Solid Edge part; units mm, degrees
sketch "Sketch1" plane through (0, 0, 0) normal (0, 0, 1) x (1, 0, 0)
  circle A0 centre (0, 0) radius 41.05
  circle A1 centre (0, 0) radius 20.625
  circle A2 centre (159.79, 0) radius 23.37
  circle A3 centre (159.79, 0) radius 13.21
extrude "Protrusion1" add sketch "Sketch1" along normal blind 17.73
sketch "Sketch2" plane through (0, 0, 0) normal (0, 0, 1) x (1, 0, 0)
  line L0 (159.79, -23.37) -> (139.6358, 0)
  line L1 (139.6358, 0) -> (159.79, 23.37)
  line L2 (8.6959, 40.1184) -> (159.79, 23.37)
  line L3 (8.6959, 40.1184) -> (28.7283, 0)
  line L4 (28.7283, 0) -> (8.6959, -40.1184)
  line L5 (159.79, -23.37) -> (8.6959, -40.1184)
extrude "ExtrudedProtrusion_2" add sketch "Sketch2" along normal blind 12.7
sketch "Sketch3" plane through (0, 0, 0) normal (0, 0, 1) x (1, 0, 0)
  line L0 (-5.0718, -15.3845) -> (-10.7875, -12.0845)
  line L1 (-10.7875, -12.0845) -> (-13.2875, -16.4147)
  line L2 (-13.2875, -16.4147) -> (-7.5718, -19.7147)
  line L3 (-5.0718, -15.3845) -> (-7.5718, -19.7147)
  line L4 (-10.7875, 12.0845) -> (-5.0718, 15.3845)
  line L5 (-5.0718, 15.3845) -> (-7.5718, 19.7147)
  line L6 (-7.5718, 19.7147) -> (-13.2875, 16.4147)
  line L7 (-10.7875, 12.0845) -> (-13.2875, 16.4147)
  line L8 (15.8593, -3.3) -> (20.8593, -3.3)
  line L9 (20.8593, -3.3) -> (20.8593, 3.3)
  line L10 (15.8593, 3.3) -> (20.8593, 3.3)
  line L11 (15.8593, 3.3) -> (15.8593, -3.3)
extrude "Protrusion2" add sketch "Sketch3" along normal up to vertex (17.73 mm away)
Verification items for the finished model (mm, model axes). A direction names the side the tool comes from. Give positions to 0.01 mm unless a question says otherwise; leave off trailing zeros. Loops run counter-clockwise (first coordinate to the right, second up) from the corner with the lowest first, then second, coordinate; pieces in that order, holes last.
1. Release check for a two-part mould opening along Y. For faces 1 (the flat face through (69, 1, 0)), 2 (the cylindrical face through (181.38, 8.95, 10.71)), 3 (the flat face through (-11.9, -14.01, 8.74)) record: +Y half, -Y half, draft (parallel to the pull), parting line (faces both ways), or undercut.
Derived:
face 1: draft
face 2: parting line
face 3: undercut
2. Material ranges on probe 1 along X at (y, z) = (-17, 14.5); probe 2 along X at (y, z) = (1.5, 11.25); probe 3 along Y at (x, z) = (159.79, 14.25), recorded low to high.
Derived:
probe 1: x = -37.36 to -6, 11.68 to 37.36, 143.75 to 175.83
probe 2: x = -41.02 to -20.57, 15.86 to 146.67, 172.91 to 183.11
probe 3: y = -23.37 to -13.21, 13.21 to 23.37
3. Cross-section at B-B on x = 0. Record the cut outline in (y, z) (3 decimals), and give its area (3 significant figures).
Derived:
outline: (-41.05, 0) - (-20.625, 0) - (-20.625, 17.73) - (-41.05, 17.73) - close; (20.625, 0) - (41.05, 0) - (41.05, 17.73) - (20.625, 17.73) - close
area: 724 mm2
4. Tool access check on faces 4 (the flat face through (85.301, -31.627, 6.261)), 5 (the flat face through (-6.181, 17.306, 8.741)), 6 (the cylindrical face through (-41, -2, 11)). Record the directions out of +Z, -Z, +X, -X, +Y, -Y that give a thin tool (end or side, any length) a straight path to the whole face; none if there is none.
Derived:
face 4: +Z, -Z, +X, -Y
face 5: +Z, -Z
face 6: +Z
5. Cross-section at C-C on y = 26. Record the cut outline in (x, z), and give its area (3 significant figures).
Derived:
outline: (-31.77, 0) - (136.06, 0) - (136.06, 12.7) - (31.77, 12.7) - (31.77, 17.73) - (-31.77, 17.73) - close
area: 2,450 mm2
6. Go/stop test with flat-tipped pins: P1, Ø6, axis at y = 19, z = 13, coming from the +X side; P2, Ø8, axis at y = -5, z = 6, coming from the -X side; P3, Ø2, axis at x = 19, z = 6, coming from the -Y side. Record where each tip stops, or that it passes through.
Derived:
P1: stops at x = 176.82
P2: stops at x = -41.04
P3: stops at y = -39.09
7. Cross-section at D-D on x = 165.5. Record the cut outline in (y, z), and give its area (3 significant figures).
Derived:
outline: (-22.66, 0) - (-11.91, 0) - (-11.91, 17.73) - (-22.66, 17.73) - close; (11.91, 0) - (22.66, 0) - (22.66, 17.73) - (11.91, 17.73) - close
area: 381 mm2
8. Cross-section at A-A on y = 0. Record the cut outline in (x, z) (3 decimals).
Derived:
outline: (-41.05, 0) - (-20.625, 0) - (-20.625, 17.73) - (-41.05, 17.73) - close; (15.859, 0) - (146.58, 0) - (146.58, 17.73) - (136.42, 17.73) - (136.42, 12.7) - (41.05, 12.7) - (41.05, 17.73) - (15.859, 17.73) - close; (173, 0) - (183.16, 0) - (183.16, 17.73) - (173, 17.73) - close
